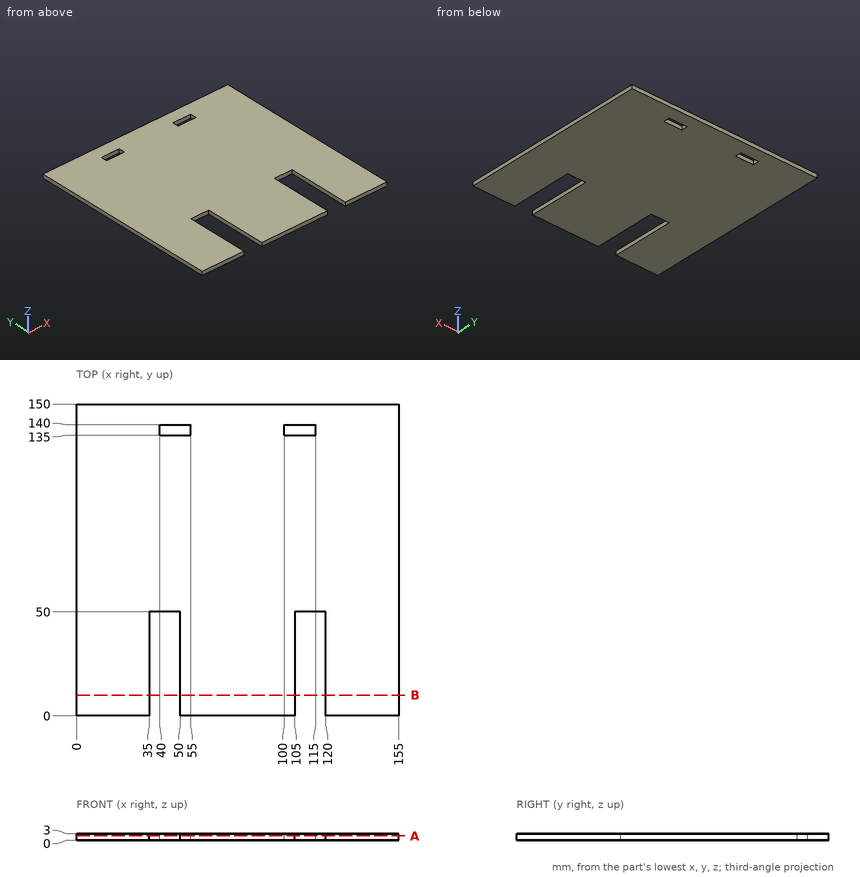
Could you check a few things on this drawing? It's one solid part, dimensions in mm from its lowest x, y, z. Coordinates: 2 decimals unless noted, no trailing zeros. Order: outer loops, then holes, each group sorted by start corner. A loop starts at its lowest first (then second) coordinate and runs counter-clockwise, first axis right, second up.
1. If we section it at B-B (y = 10): Please give me the cut outline in (x, z).
2. I need wall thicknesses on line 1 (X direction, y = 23, z = 0.8); line 2 (X direction, y = 139.5, z = 0.4); line 3 (Y direction, x = 52.5, z = 2.5). Which ranges of each line are inside material? Lowest first, please.
3. If we section it at A-A (z = 2): Please give me the cut outline in (x, y).
4. I'm going to push flat-ended pins straight in: pin 1 (1.5 mm diameter, centred on y = 14, z = 1, fed in from -X); pin 2 (1.5 mm diameter, centred on x = 48, z = 1, fed in from -Y). Where does each tip first touch, or does it pass through?
Entries:
1. outline: (0, 0) - (35, 0) - (35, 3) - (0, 3) - close; (50, 0) - (105, 0) - (105, 3) - (50, 3) - close; (120, 0) - (155, 0) - (155, 3) - (120, 3) - close
2. line 1: x = 0 to 35, 50 to 105, 120 to 155
2. line 2: x = 0 to 40, 55 to 100, 115 to 155
2. line 3: y = 0 to 135, 140 to 150
3. outline: (0, 0) - (35, 0) - (35, 50) - (50, 50) - (50, 0) - (105, 0) - (105, 50) - (120, 50) - (120, 0) - (155, 0) - (155, 150) - (0, 150) - close; hole (40, 135) - (55, 135) - (55, 140) - (40, 140) - close; hole (100, 135) - (115, 135) - (115, 140) - (100, 140) - close
4. pin 1: stops at x = 0
4. pin 2: stops at y = 50
